Can you work these out from the drawing? Everything is in mm from the part's minimum corner. A direction names the side the tool comes from. Round coordinates to 2 decimals unless told otherwise and drop trailing zeros. Loops run counter-clockwise (first coordinate to the right, second up) from the corner with the lowest first, then second, coordinate; pieces in that order, holes last. Notation, with made-up numbers: (11, -4) -> (51, -4) arc R23 ccw to (51, 21) -> close; hole circle Ø5 at (36, 29). An arc over 180 degrees is marked (long way). One line per item, written item: value.
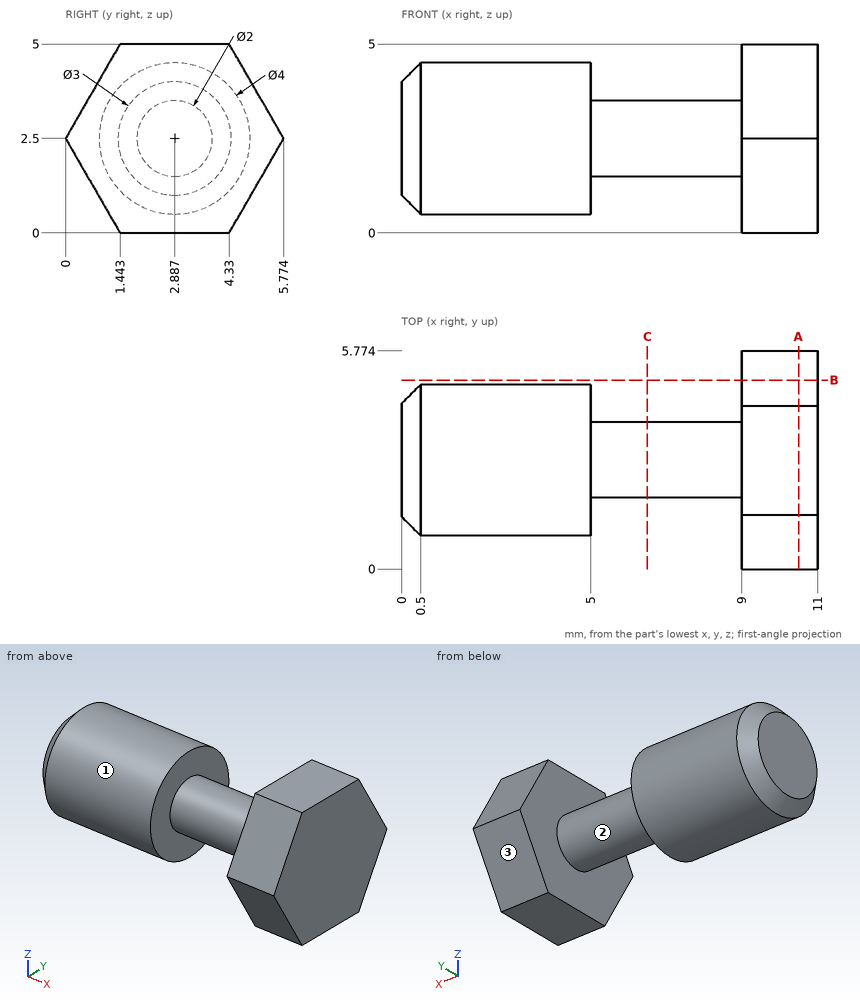
Item 1: I need wall thicknesses on line 1 (X direction, y = 3.6, z = 1.2); line 2 (Z direction, x = 8.5, y = 2.95); line 3 (X direction, y = 1.45, z = 4.75). Which ranges of each line are inside material? Lowest first, please. Write a range as from..to.
Output:
line 1: x = 0..5, 9..11
line 2: z = 1.5..3.5
line 3: x = 9..11
Item 2: If we section it at A-A on x = 10.5: List the corners of the cut face in (y, z) for me.
Output:
outline: (0, 2.5) -> (1.44, 0) -> (4.33, 0) -> (5.77, 2.5) -> (4.33, 5) -> (1.44, 5) -> close
Item 3: If we section it at C-C on x = 6.5: List the corners of the cut face in (y, z) for me.
Output:
outline: circle Ø2 at (2.89, 2.5)
Item 4: For the marked faces 1, 2 and 3, which set-ups out of +Z, -Z, +X, -X, +Y, -Y let a thin tool reach every point of the face, with its end or its side?
Output:
face 1: -X
face 2: none
face 3: -Z, +X, -X, +Y
Item 5: If we section it at B-B on y = 5: List the corners of the cut face in (x, z) for me.
Output:
outline: (9, 1.16) -> (11, 1.16) -> (11, 3.84) -> (9, 3.84) -> close
Item 6: Will these pins go through, and if not, where does the flat tip stop? pin 1 Ø1 at (x, z) = (9, 3.5) entering from -Y; pin 2 Ø1.5 at (x, y) = (7, 3.5) entering from -Z.
Output:
pin 1: stops at y = 0.29
pin 2: stops at z = 1.5
